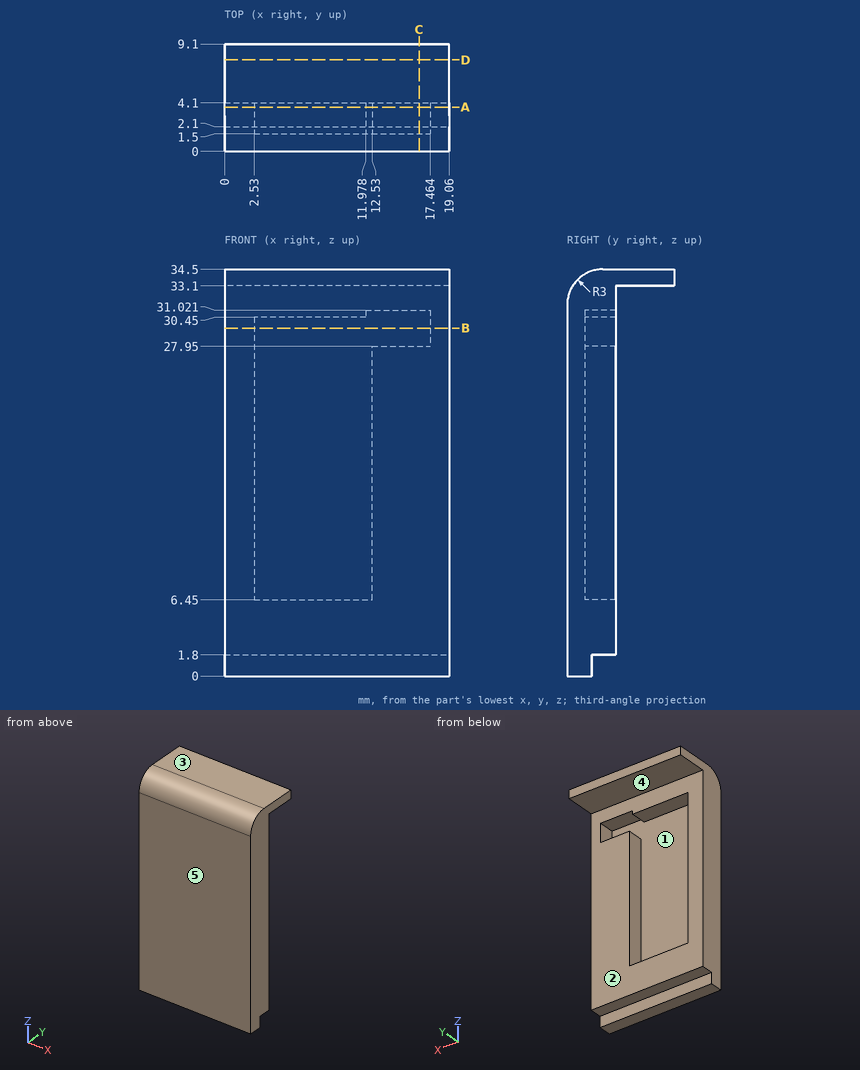
Print and shaded views of the part. All mm, measured from the part's lowest x, y and z. A direction names the side the tool comes from. Coordinates: 2 decimals unless noted, no trailing zeros. Loops run counter-clockwise (first coordinate to the right, second up) from the corner with the lowest first, then second, coordinate; pieces in that order, holes last. Notation, with made-up numbers: (44, 88) - (64, 88) arc R14 cw to (64, 113) - close; hole circle Ø11 at (-36, 8). An arc over 180 degrees is marked (long way). Write item = value, one per line. Start each with the question number.
Item 1: Saw through at C-C, the plane x = 16.5. List the corners of the cut face in (y, z), then the cut area to 3 significant figures.
Item 2: Pull direction Z, two halves, no side cores. Call the marked faces 1, 2 and 3: +Z half, -Z half, draft (parallel to the pull), parting line (faces both ways), or undercut.
Item 3: Saw through at D-D, the plane y = 7.75. List the corners of the cut face in (x, z), then the cut area to 3 significant figures.
Item 4: Saw through at B-B, the plane z = 29.5. List the corners of the cut face in (x, y), then the cut area to 3 significant figures.
Item 5: Wall check: probe 1 along Z at (x, y) = (4, 4); probe 2 along X at (y, z) = (3.25, 7); probe 3 along Y at (x, z) = (9.25, 17). Give the ranges that are in metal, low to high. Write a range as [from, to].
Item 6: Saw through at A-A, the plane y = 3.75. List the corners of the cut face in (x, z), then the cut area to 3 significant figures.
Item 7: Drop flat-ended pins along their axis: pin 1 Ø4.5 at (x, z) = (8, 15) entering from +Y; pin 2 Ø10 at (x, z) = (9.5, 21.5) entering from +Y; pin 3 Ø0.5 at (x, z) = (8, 1) entering from +Y. Give the stop position or say it passes through.
Item 8: 3-axis set-ups, long thin cutter, end or side, ignore diameter. For the marked faces 4 and 5: which of +Z, -Z, +X, -X, +Y, -Y reach the whole face in a straight line?
Answers:
q1.outline = (0, 0) - (2.1, 0) - (2.1, 1.8) - (4.1, 1.8) - (4.1, 27.95) - (1.5, 27.95) - (1.5, 31.02) - (4.1, 31.02) - (4.1, 33.1) - (9.1, 33.1) - (9.1, 34.5) - (3, 34.5) arc R3 ccw to (0, 31.5) - close
q1.area = 135 mm2
q2.face_1 = undercut
q2.face_2 = draft
q2.face_3 = +Z half
q3.outline = (0, 33.1) - (19.06, 33.1) - (19.06, 34.5) - (0, 34.5) - close
q3.area = 26.7 mm2
q4.outline = (0, 0) - (19.06, 0) - (19.06, 4.1) - (17.46, 4.1) - (17.46, 1.5) - (2.53, 1.5) - (2.53, 4.1) - (0, 4.1) - close
q4.area = 39.3 mm2
q5.probe_1 = [1.8, 6.45], [30.45, 34.5]
q5.probe_2 = [0, 2.53], [12.53, 19.06]
q5.probe_3 = [0, 1.5]
q6.outline = (0, 1.8) - (19.06, 1.8) - (19.06, 34.5) - (0, 34.5) - close; hole (2.53, 6.45) - (12.53, 6.45) - (12.53, 27.95) - (17.46, 27.95) - (17.46, 31.02) - (11.98, 31.02) - (11.98, 30.45) - (2.53, 30.45) - close
q6.area = 368 mm2
q7.pin_1 = 1.5
q7.pin_2 = 4.1
q7.pin_3 = 2.1
q8.face_4 = -Z, +X, -X, +Y
q8.face_5 = +Z, -Z, +X, -X, -Y
